```python
from build123d import *

# Parameters (mm, degrees)
F2_R     = 11.25
F0_DEPTH = 3.15
F3_R     = 1.414991
F4_DEPTH = 3.15
F5_DEPTH = 1


with BuildPart() as f0:
    # F2 (on Top) → F0 (new body)
    with BuildSketch(Plane.XY):
        Circle(F2_R)
    extrude(amount=F0_DEPTH)

    # F3 (on face) → F4 (cut, through all)
    with BuildSketch(Plane.XY.offset(3.15)):
        with Locations((0, 8.5)):
            Circle(F3_R)
    extrude(amount=-F4_DEPTH, mode=Mode.SUBTRACT)

    # F1 (on face) → F5 (cut)
    with BuildSketch(Plane.XY.offset(3.15)):
        with BuildLine():
            ThreePointArc((0, 0), (-2, 2), (-4, 0))
            ThreePointArc((-4, 0), (-2.62543, -3.587054), (0, -6.391252))
            ThreePointArc((0, -6.391252), (2.62543, -3.587054), (4, 0))
            ThreePointArc((4, 0), (2, 2), (0, 0))
        make_face()
    extrude(amount=-F5_DEPTH, mode=Mode.SUBTRACT)


solid = f0.part
```
Design review of the part built by this model. Coordinates are the model's own, in mm. A direction names the side the tool comes from. Coordinates: 2 decimals unless noted, no trailing zeros. Loops run counter-clockwise (first coordinate to the right, second up) from the corner with the lowest first, then second, coordinate; pieces in that order, holes last. Notation, with made-up numbers: (-28, 67) -> (27, 67) arc R22 cw to (27, 102) -> close; hole circle Ø6 at (-35.75, -23). An arc over 180 degrees is marked (long way). Answer as a JSON object with one key per item and string values.
Q1. Clearance check with flat-ended pins moving along their axes: pin 1 Ø1.5 at (x, z) = (-2.5, 2) entering from +Y; pin 2 Ø2.5 at (x, y) = (0, 8.5) entering from +Z; pin 3 Ø1.5 at (y, z) = (1, 2.5) entering from +X; pin 4 Ø1 at (x, z) = (-1.5, 2.5) entering from -Y. State where each tip first meets the part, or that it passes through.
Answer block:
{"pin 1": "stops at y = 11.11", "pin 2": "passes through", "pin 3": "stops at x = 11.25", "pin 4": "stops at y = -11.21"}
Q2. Take a section at D-D on y = 8.5. Give the boundary of the cut face in (x, z) (3 decimals).
Answer block:
{"outline": "(-7.37, 0) -> (-1.415, 0) -> (-1.415, 3.15) -> (-7.37, 3.15) -> close; (1.415, 0) -> (7.37, 0) -> (7.37, 3.15) -> (1.415, 3.15) -> close"}
Q3. Take a section at B-B on z = 0.7. Give the boundary of the cut face in (x, y) (3 decimals), plus the area to 3 significant figures.
Answer block:
{"outline": "circle Ø22.5 at (0, 0); hole circle Ø2.83 at (0, 8.5)", "area": "391 mm^2"}
Q4. The part is to be moulded in two halves that separate along Y. For faces 1 (the cylindrical face through (-0.31, 7.12, 1.6)), 2 (the cylindrical face through (5.19, -9.98, 1.55)), 3 (the flat face through (0, 0, 0)), say which applies: +Y half, -Y half, draft (parallel to the pull), parting line (faces both ways), or undercut.
Answer block:
{"face 1": "undercut", "face 2": "parting line", "face 3": "draft"}
Q5. Tool access review of faces 4 (the flat face through (0, 3, 3.15)), 5 (the flat face through (0, -1, 2.15)): name each direction out of +Z, -Z, +X, -X, +Y, -Y from which nothing blocks a thin tool from reaching the whole face with its end or side.
Answer block:
{"face 4": "+Z, +X, -X, +Y, -Y", "face 5": "+Z"}
Q6. Take a section at C-C on z = 2.7. Give the boundary of the cut face in (x, y) (3 decimals), plus the area to 3 significant figures.
Answer block:
{"outline": "circle Ø22.5 at (0, 0); hole (-4, 0) arc R10 ccw to (0, -6.391) arc R10 ccw to (4, 0) arc R2 ccw to (0, 0) arc R2 ccw to start; hole circle Ø2.83 at (0, 8.5)", "area": "346 mm^2"}
Q7. To check wall thickness, follow L1, parallel to Y at x = 0, z = 0.7 (3 decimals); L2, parallel to X at y = 8, z = 0.75; L3, parallel to Y at x = -4, z = 1.6. State the ranges of each line that lie inside material, in increasing order.
Answer block:
{"L1": "y = -11.25 to 7.085, 9.915 to 11.25", "L2": "x = -7.91 to -1.32, 1.32 to 7.91", "L3": "y = -10.51 to 10.51"}
Q8. Take a section at A-A on x = 0.5. Give the boundary of the cut face in (y, z).
Answer block:
{"outline": "(-11.24, 0) -> (7.18, 0) -> (7.18, 3.15) -> (1.32, 3.15) -> (1.32, 2.15) -> (-6.01, 2.15) -> (-6.01, 3.15) -> (-11.24, 3.15) -> close; (9.82, 0) -> (11.24, 0) -> (11.24, 3.15) -> (9.82, 3.15) -> close"}
